Part print with two shaded views. Sizes in mm from the minimum x, y, z corner. A direction names the side the tool comes from. Coordinates: 2 decimals unless noted, no trailing zeros. Loops run counter-clockwise (first coordinate to the right, second up) from the corner with the lowest first, then second, coordinate; pieces in that order, holes last.
Item 1: 3-axis set-ups, long thin cutter, end or side, ignore diameter. For the marked faces 1, 2 and 3: which of +Z, -Z, +X, -X, +Y, -Y reach the whole face in a straight line?
Item 2: Drill centre lines: line 1 along Z through (x, y) = (23.85, 2.35); line 2 along X through (y, z) = (3, 36.65); line 3 along Z through (x, y) = (25, 2.5). Where is each one in solid material? Low to high.
Item 3: Cut at C-C (y = 3.45). Count the separate pieces of the cut face and the enclosed holes in it, and give its area (3 significant figures).
Item 4: Cut at B-B (z = 21.15). List the corners of the cut face in (x, y), and give its area (4 significant figures).
Item 5: Cut at D-D (x = 23.85). List the corners of the cut face in (y, z), and give its area (4 significant figures).
Item 6: Mould opens along Z. For the marked faces 4, 5 and 6 say: released by +Z, released by -Z, zero draft, split by the parting line, or undercut.
Item 7: Cut at A-A (x = 39.35). List the corners of the cut face in (y, z).
Item 8: Flat gauge pins, fed straight in: pin 1 (1 mm diameter, centred on x = 77, y = 2, fed in from +Z); pin 2 (2 mm diameter, centred on y = 1.5, z = 38, fed in from -X); pin 3 (3 mm diameter, centred on y = 3.5, z = 19, fed in from -X); pin 4 (1.2 mm diameter, centred on y = 1.5, z = 37.5, fed in from +X). Where does each tip first touch, or does it go through?
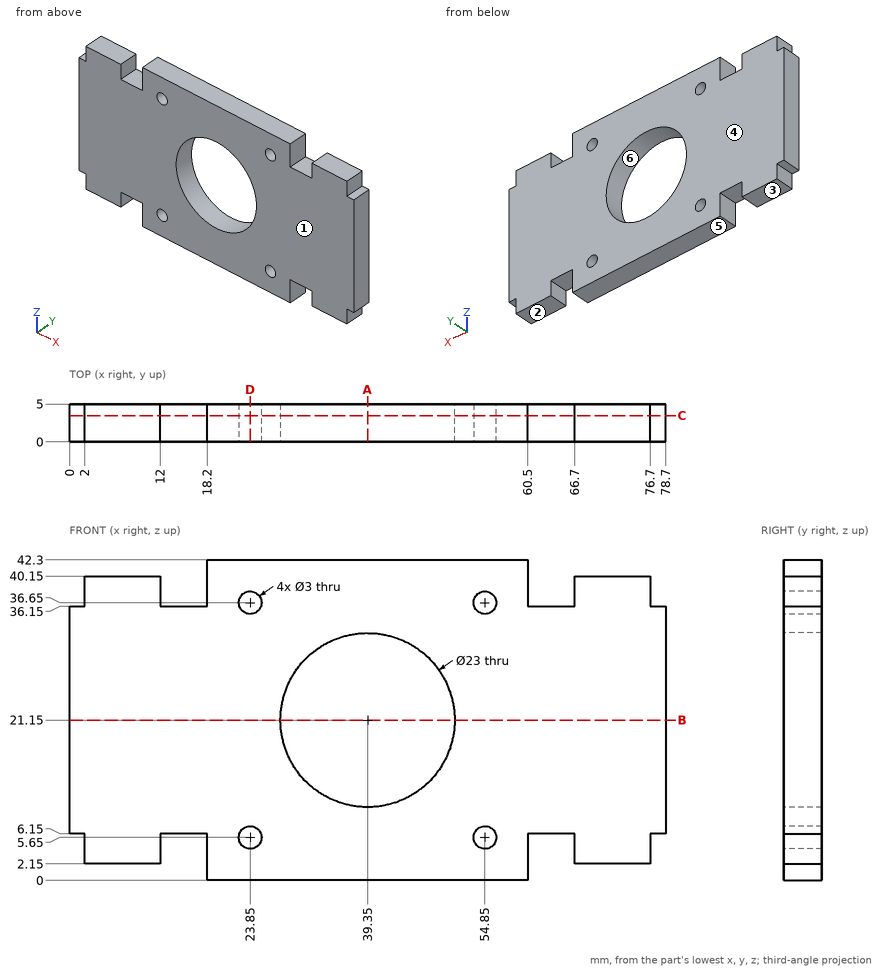
Filled sheet:
1. face 1: +Z, -Z, +X, -X, -Y
1. face 2: -Z, +X, +Y, -Y
1. face 3: -Z, -X, +Y, -Y
2. line 1: z = 0 to 4.15, 7.15 to 35.15, 38.15 to 42.3
2. line 2: x = 2 to 12, 18.2 to 22.35, 25.35 to 53.35, 56.35 to 60.5, 66.7 to 76.7
2. line 3: z = 0 to 4.69, 6.61 to 35.69, 37.61 to 42.3
3. separate pieces: 1
3. enclosed holes: 5
3. area: 2,600 mm2
4. outline: (0, 0) - (27.85, 0) - (27.85, 5) - (0, 5) - close; (50.85, 0) - (78.7, 0) - (78.7, 5) - (50.85, 5) - close
4. area: 278.5 mm2
5. outline: (0, 0) - (5, 0) - (5, 4.15) - (0, 4.15) - close; (0, 7.15) - (5, 7.15) - (5, 35.15) - (0, 35.15) - close; (0, 38.15) - (5, 38.15) - (5, 42.3) - (0, 42.3) - close
5. area: 181.5 mm2
6. face 4: zero draft
6. face 5: released by -Z
6. face 6: undercut
7. outline: (0, 0) - (5, 0) - (5, 9.65) - (0, 9.65) - close; (0, 32.65) - (5, 32.65) - (5, 42.3) - (0, 42.3) - close
8. pin 1: stops at z = 40.15
8. pin 2: stops at x = 2
8. pin 3: stops at x = 0
8. pin 4: stops at x = 76.7
